Check sheet for the drawn part. Datum: minimum x, y, z corner. Units: mm. Give positions to 0.01 mm unless a question says otherwise; leave off trailing zeros. Order: outer loops, then holes, each group sorted by start corner. A loop starts at its lowest first (then second) coordinate and runs counter-clockwise, first axis right, second up. Notation, with made-up numbers: M 59,46 L 71,46 A26 ccw 71,61 Z; hole C 9,27.5 d5. An arc over 180 degrees is marked long. Put each result on its own line as item: value. Start each with the question number.
Q1. Section check C-C on z = 24. Record the cut outline in (x, y).
Q2. Mould release check, pull along X, two halves, no side actions. Record for the marked faces 1 and 2: +X half, -X half, draft (parallel to the pull), parting line (faces both ways), or undercut.
Q3. Go/stop test with flat-tipped pins: pin 1 (1.5 mm diameter, centred on x = 1, z = 64.5, fed in from -Y); pin 2 (4 mm diameter, centred on y = 15.5, z = 17.5, fed in from -X). Record where each tip stops, or that it passes through.
Q4. Section check A-A on y = 7.5. Record the cut outline in (x, z), then the cut area to 3 significant figures.
Q5. Section check B-B on x = 1.9. Record the cut outline in (y, z), then the cut area to 3 significant figures.
Q6. Material ranges on L1, parallel to Y at x = 1.75, z = 92.5; L2, parallel to Y at x = 2.2, z = 11, recorded low to high.
Q7. Section check D-D on z = 99.5. Record the cut outline in (x, y), then the cut area to 3 significant figures.
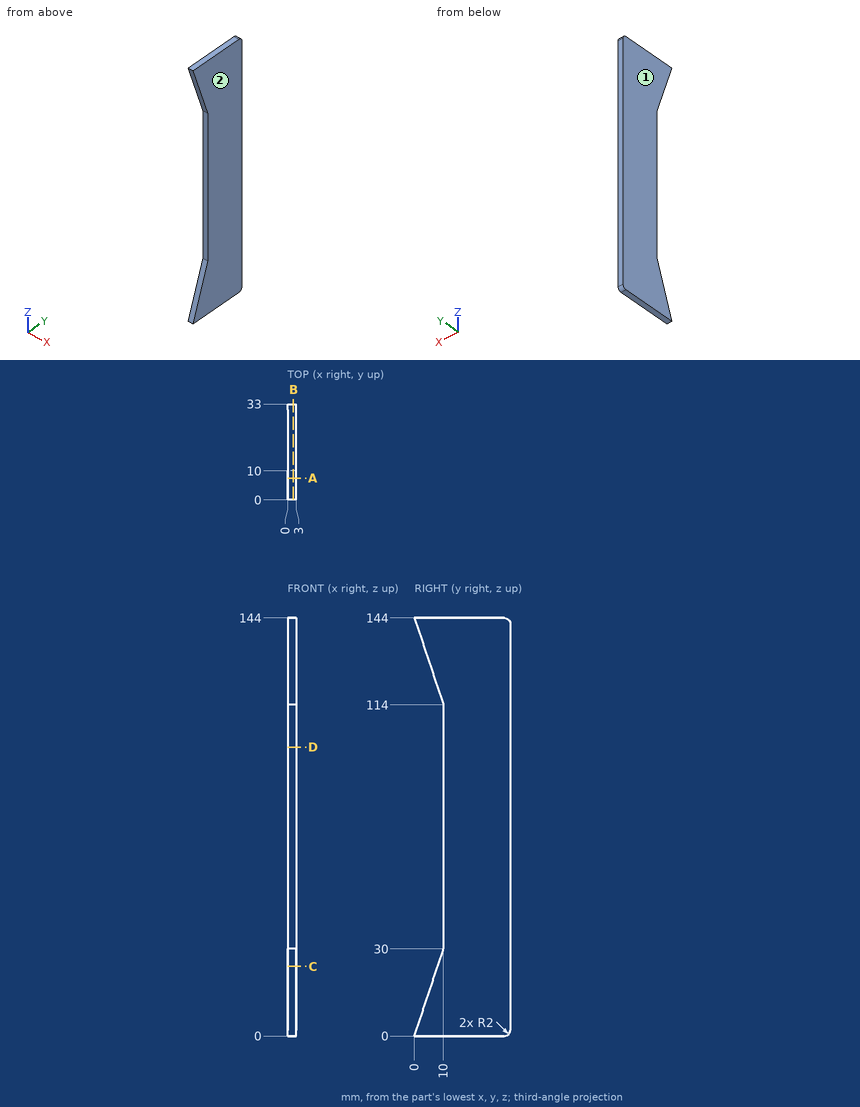
Results found:
1. outline: M 0,8 L 3,8 L 3,33 L 0,33 Z
2. face 1: -X half
2. face 2: +X half
3. pin 1: stops at y = 10
3. pin 2: stops at x = 0
4. outline: M 0,0 L 3,0 L 3,22.5 L 0,22.5 Z; M 0,121.5 L 3,121.5 L 3,144 L 0,144 Z
4. area: 135 mm^2
5. outline: M 0,0 L 31,0 A2 ccw 33,2 L 33,142 A2 ccw 31,144 L 0,144 L 10,114 L 10,30 Z
5. area: 3,610 mm^2
6. L1: y = 10 to 33
6. L2: y = 3.67 to 33
7. outline: M 0,10 L 3,10 L 3,33 L 0,33 Z
7. area: 69.0 mm^2
